Print and shaded views of the part. All mm, measured from the part's lowest x, y and z. Round coordinates to 2 decimals unless told otherwise and drop trailing zeros. Order: outer loops, then holes, each group sorted by start corner. A loop starts at its lowest first (then second) coordinate and runs counter-clockwise, first axis right, second up. Notation, with made-up numbers: (44, 71) -> (103, 71) arc R12 cw to (103, 81) -> close; hole circle Ø4 at (30, 89.5). An arc over 180 degrees is marked (long way). Answer as CSV lines item,"result".
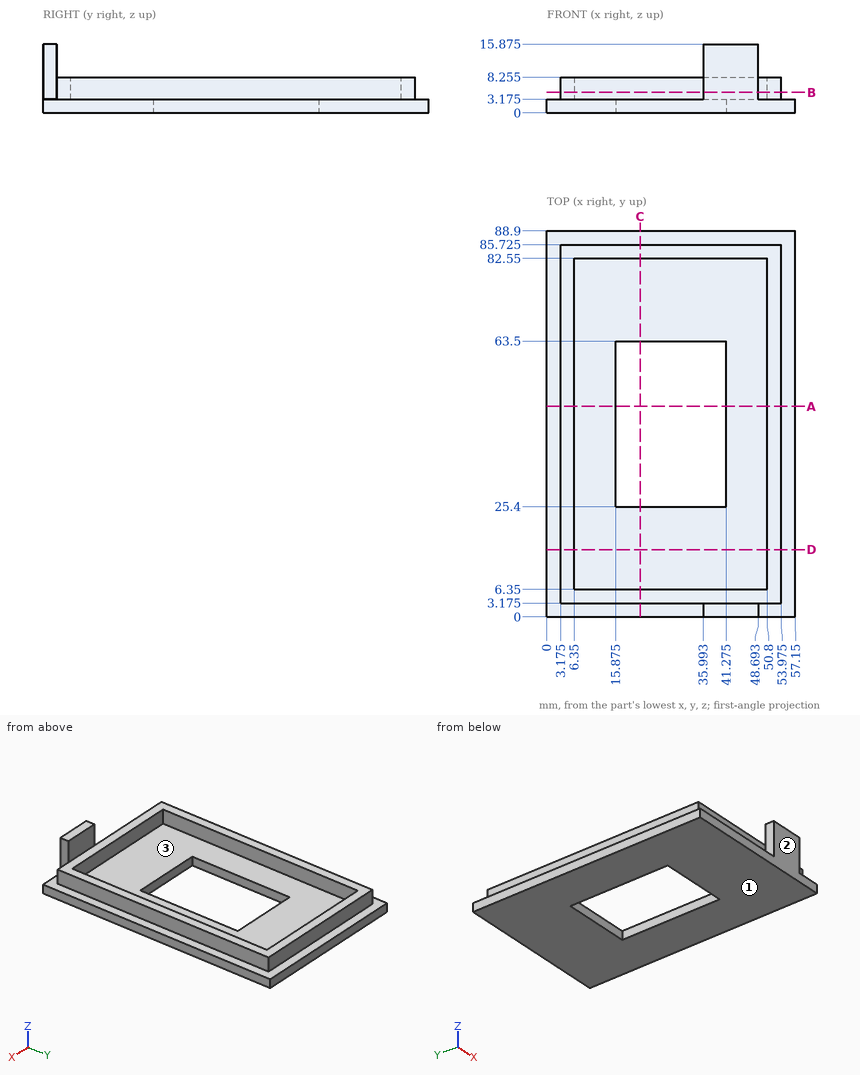
Q1. Saw through at C-C (x = 21.5). Write the cut outline in (y, z) (3 decimals).
Checks:
outline,"(0, 0) -> (25.4, 0) -> (25.4, 3.175) -> (6.35, 3.175) -> (6.35, 8.255) -> (3.175, 8.255) -> (3.175, 3.175) -> (0, 3.175) -> close; (63.5, 0) -> (88.9, 0) -> (88.9, 3.175) -> (85.725, 3.175) -> (85.725, 8.255) -> (82.55, 8.255) -> (82.55, 3.175) -> (63.5, 3.175) -> close"
Q2. Saw through at D-D (y = 15.5). Write the cut outline in (x, z) (3 decimals), plus the area to 3 significant figures.
Checks:
outline,"(0, 0) -> (57.15, 0) -> (57.15, 3.175) -> (53.975, 3.175) -> (53.975, 8.255) -> (50.8, 8.255) -> (50.8, 3.175) -> (6.35, 3.175) -> (6.35, 8.255) -> (3.175, 8.255) -> (3.175, 3.175) -> (0, 3.175) -> close"
area,"214 mm²"
Q3. Saw through at B-B (z = 4.75). Write the cut outline in (x, y) (3 decimals), plus the area to 3 significant figures.
Checks:
outline,"(3.175, 3.175) -> (35.993, 3.175) -> (35.993, 0) -> (48.693, 0) -> (48.693, 3.175) -> (53.975, 3.175) -> (53.975, 85.725) -> (3.175, 85.725) -> close; hole (6.35, 6.35) -> (50.8, 6.35) -> (50.8, 82.55) -> (6.35, 82.55) -> close"
area,"847 mm²"
Q4. Saw through at A-A (y = 48.5). Write the cut outline in (x, z) (3 decimals).
Checks:
outline,"(0, 0) -> (15.875, 0) -> (15.875, 3.175) -> (6.35, 3.175) -> (6.35, 8.255) -> (3.175, 8.255) -> (3.175, 3.175) -> (0, 3.175) -> close; (41.275, 0) -> (57.15, 0) -> (57.15, 3.175) -> (53.975, 3.175) -> (53.975, 8.255) -> (50.8, 8.255) -> (50.8, 3.175) -> (41.275, 3.175) -> close"
Q5. Mould opens along Y. For the marked faces 1, 2 and 3 say: +Y half, -Y half, draft (parallel to the pull), parting line (faces both ways), or undercut.
Checks:
face 1,"draft"
face 2,"-Y half"
face 3,"undercut"
Q6. Wall check: L1, parallel to Y at x = 43.5, z = 6.25 (3 decimals); L2, parallel to X at y = 38, z = 3 (3 decimals); L3, parallel to Y at x = 7, z = 3.25 (3 decimals). Give the ranges that are in metal, low to high. Write a range as [from, to].
Checks:
L1,"[0, 6.35], [82.55, 85.725]"
L2,"[0, 15.875], [41.275, 57.15]"
L3,"[3.175, 6.35], [82.55, 85.725]"
Q7. Flat gauge pins, fed straight in: pin 1 (1.5 mm diameter, centred on x = 19, z = 6, fed in from -Y) (3 decimals); pin 2 (1.5 mm diameter, centred on y = 57, z = 5.5, fed in from +X) (3 decimals); pin 3 (6 mm diameter, centred on x = 23.5, z = 9.5, fed in from +Y) (3 decimals). Where does each tip first touch, or does it go through?
Checks:
pin 1,"y = 3.175"
pin 2,"x = 53.975"
pin 3,"y = 85.725"
